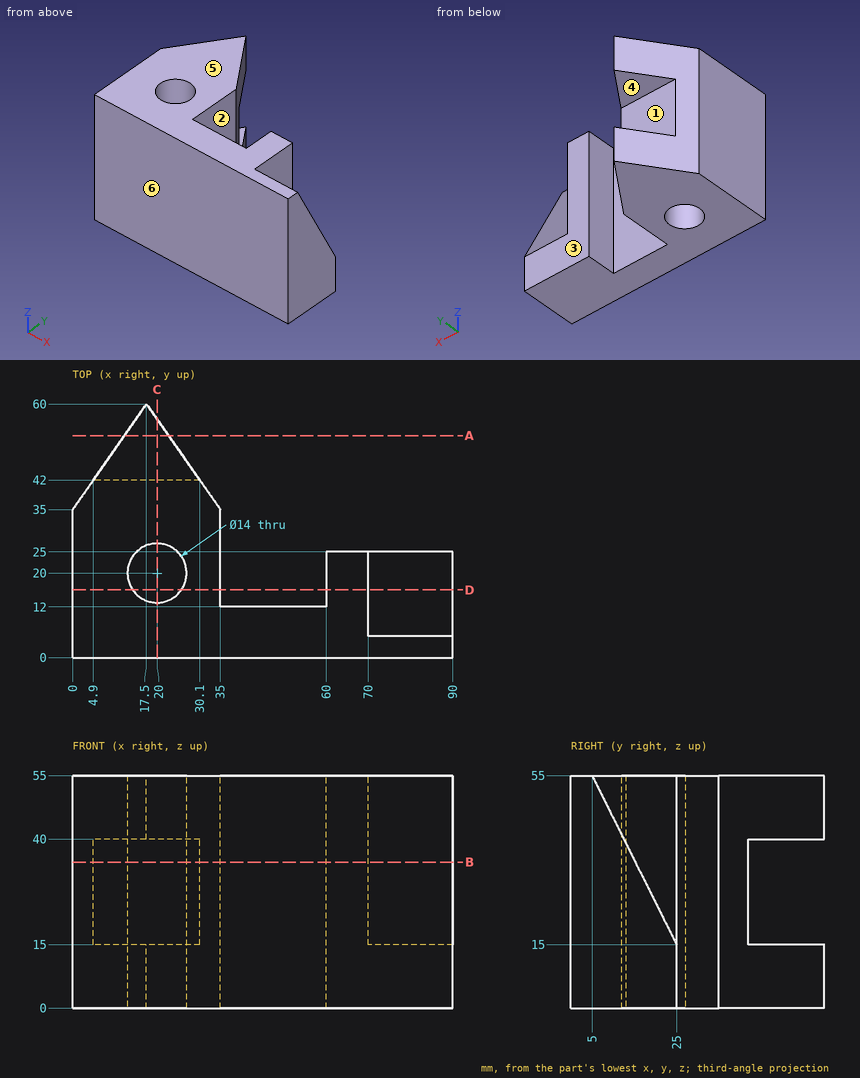
The figure shows three views and two pictorial views of one solid part (mm, origin at its lowest corner). Answer the questions. A direction names the side the tool comes from. Give positions to 0.01 mm unless a question says otherwise; leave off trailing zeros. Write each loop counter-clockwise with the first axis right and the second up, starting at its lowest first coordinate (ties: lowest second). Pieces come first, ordered by that corner, then holes. Notation, with made-up numbers: (6.25, 87.5) - (62.25, 87.5) arc R15 ccw to (62.25, 98.5) - close; hole circle Ø1 at (-37.75, -12). An arc over 180 degrees is marked (long way). Use one line per item in the form item = value.
1. A cutting plane is placed at D-D (y = 16). Write down the section's boundary in (x, z).
Filled in:
outline = (0, 0) - (14.26, 0) - (14.26, 55) - (0, 55) - close; (25.74, 0) - (35, 0) - (35, 55) - (25.74, 55) - close; (60, 0) - (90, 0) - (90, 33) - (70, 33) - (70, 55) - (60, 55) - close
2. A cutting plane is placed at A-A (y = 52.5). Write down the section's boundary in (x, z), and give its area (3 significant figures).
Filled in:
outline = (12.25, 0) - (22.75, 0) - (22.75, 15) - (12.25, 15) - close; (12.25, 40) - (22.75, 40) - (22.75, 55) - (12.25, 55) - close
area = 315 mm^2
3. A cutting plane is placed at C-C (x = 20). Write down the section's boundary in (y, z).
Filled in:
outline = (0, 0) - (13, 0) - (13, 55) - (0, 55) - close; (27, 0) - (56.43, 0) - (56.43, 15) - (42, 15) - (42, 40) - (56.43, 40) - (56.43, 55) - (27, 55) - close
4. A cutting plane is placed at B-B (z = 34.5). Write down the section's boundary in (x, y).
Filled in:
outline = (0, 0) - (90, 0) - (90, 15.25) - (70, 15.25) - (70, 25) - (60, 25) - (60, 12) - (35, 12) - (35, 35) - (30.1, 42) - (4.9, 42) - (0, 35) - close; hole circle Ø14 at (20, 20)
5. Determine the mould class of the marked faces 4, 5 and 6 for opening direction Z: released by +Z, released by -Z, zero draft, split by the parting line, or undercut.
Filled in:
face_4 = undercut
face_5 = released by +Z
face_6 = zero draft
6. Consider L1, parallel to Y at x = 20, z = 24.5; L2, parallel to X at y = 22, z = 17; L3, parallel to Z at x = 16, y = 44.5. Determine where each line is inside the solid, lowest interval first.
Filled in:
L1 = 0 to 13, 27 to 42
L2 = 0 to 13.29, 26.71 to 35, 60 to 90
L3 = 0 to 15, 40 to 55
7. For the marked faces 1, 2 and 3, determine the directions among +Z, -Z, +X, -X, +Y, -Y from which every point of the face is accessible in a straight line to the end or side of a thin tool.
Filled in:
face_1 = +X, -X, +Y
face_2 = +Z, -Z, +Y
face_3 = +Z, -Z, +X, +Y
8. Each of these flat-tipped pins is pushed along its axis until it touches: pin 1 Ø1.5 at (x, z) = (74, 16) entering from +Y (3 decimals); pin 2 Ø11 at (x, y) = (20, 20) entering from +Z (3 decimals); pin 3 Ø7 at (y, z) = (21, 39) entering from +X; pin 4 Ø15 at (x, z) = (69.5, 15) entering from +Y. Where does it stop, or does it pass through?
Filled in:
pin_1 = 24.875
pin_2 = through
pin_3 = 70
pin_4 = 25
